Build history of the part. All positions in model axes, mm. Face numbers are marked on the shaded views. A direction names the side the tool comes from. Give positions to 0.01 mm unless a question says otherwise; leave off trailing zeros. Order: outer loops, then holes, each group sorted by start corner. A loop starts at its lowest first (then second) coordinate and runs counter-clockwise, first axis right, second up. Notation, with made-up numbers: (69, 32.5) -> (111, 32.5) arc R23 cw to (111, 48.5) -> close; hole circle Ø5 at (-25.75, -29). An arc over 180 degrees is marked (long way). One line per item, written item: value. Start each with the question number.
(1) Saw through at D-D on z = 5.25. Give the cut face in (x, y).
(2) Which spindle directions (+Z, -Z, +X, -X, +Y, -Y) get a long thin tool onto all of the face, cutting with end or side? Do the marked faces 5, 6, 7 and 8. Say none if no direction does.
(3) Saw through at C-C on z = -3. Give the cut face in (x, y), plus the area to 3 significant figures.
(4) Saw through at A-A on y = 0. Give the cut face in (x, z).
(5) Two-plate mould, pull along Y, no slides. Class the marked faces 1, 2, 3 and 4: +Y half, -Y half, draft (parallel to the pull), parting line (faces both ways), or undercut.
(6) Saw through at B-B on x = 0. Give the cut face in (y, z).
(7) Pin check, flat tips, straight feed: pin 1 (4 mm diameter, centred on y = 17, z = 5.5, fed in from -X); pin 2 (1.5 mm diameter, centred on x = 1, z = 6, fed in from +Y); pin 3 (1 mm diameter, centred on y = -15.5, z = -2.5, fed in from -X). Stop position of each tip, or through.
(8) Probe line 1 (X direction, y = -1, z = 5); line 2 (Y direction, x = 0, z = -0.75); line 3 (Z direction, x = -12.5, y = -17.5). List the from-to ranges inside material, lowest first.
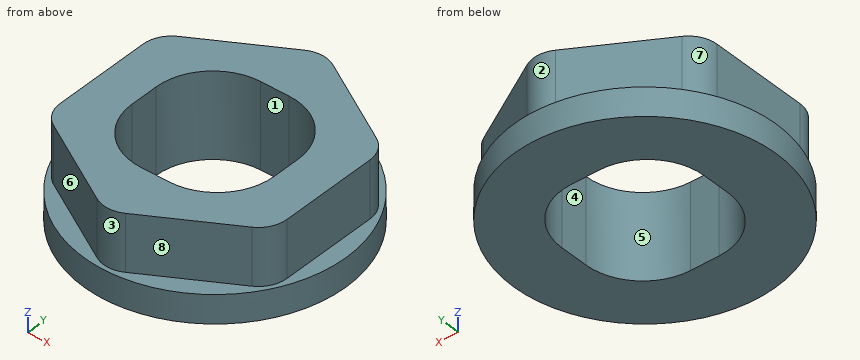
```python
from build123d import *

# Parameters (mm, degrees)
BOSS_EXTRUDE1_DEPTH = 10
SKETCH2_R           = 23.094010768
BOSS_EXTRUDE2_DEPTH = 5
FILLET1_R           = 5


with BuildPart() as part:
    # Sketch1 → Boss-Extrude1 (new body)
    with BuildSketch(Plane.XY):
        Polygon((20, -11.547005384), (20, 11.547005384), (0, 23.094010768), (-20, 11.547005384), (-20, -11.547005384), (0, -23.094010768), align=None)
        with BuildLine():
            Line((2.5, -12.5), (-2.5, -12.5))
            ThreePointArc((-2.5, -12.5), (-9.571067812, -9.571067812), (-12.5, -2.5))
            Line((-12.5, -2.5), (-12.5, 2.5))
            ThreePointArc((-12.5, 2.5), (-9.571067812, 9.571067812), (-2.5, 12.5))
            Line((-2.5, 12.5), (2.5, 12.5))
            ThreePointArc((2.5, 12.5), (9.571067812, 9.571067812), (12.5, 2.5))
            Line((12.5, 2.5), (12.5, -2.5))
            ThreePointArc((12.5, -2.5), (9.571067812, -9.571067812), (2.5, -12.5))
        make_face(mode=Mode.SUBTRACT)
    extrude(amount=BOSS_EXTRUDE1_DEPTH)

    # Sketch2 → Boss-Extrude2 (add)
    with BuildSketch(Plane(origin=(0, 0, 0), x_dir=(-1, 0, 0), z_dir=(0, 0, -1))):
        Circle(SKETCH2_R)
        with BuildLine():
            Line((-2.5, 12.5), (2.5, 12.5))
            ThreePointArc((2.5, 12.5), (9.571067812, 9.571067812), (12.5, 2.5))
            Line((12.5, 2.5), (12.5, -2.5))
            ThreePointArc((12.5, -2.5), (9.571067812, -9.571067812), (2.5, -12.5))
            Line((2.5, -12.5), (-2.5, -12.5))
            ThreePointArc((-2.5, -12.5), (-9.571067812, -9.571067812), (-12.5, -2.5))
            Line((-12.5, -2.5), (-12.5, 2.5))
            ThreePointArc((-12.5, 2.5), (-9.571067812, 9.571067812), (-2.5, 12.5))
        make_face(mode=Mode.SUBTRACT)
    extrude(amount=BOSS_EXTRUDE2_DEPTH)

    # Fillet1
    fillet1_edges = [part.edges().sort_by_distance(p)[0] for p in [
        (20, -11.547005384, 5),
        (0, -23.094010768, 5),
        (-20, -11.547005384, 5),
        (-20, 11.547005384, 5),
        (0, 23.094010768, 5),
        (20, 11.547005384, 5),
    ]]
    fillet(fillet1_edges, radius=FILLET1_R)


solid = part.part
```
Results below:
1. outline: (-20, -8.66) arc R5 ccw to (-17.5, -12.99) -> (-2.5, -21.65) arc R5 ccw to (2.5, -21.65) -> (17.5, -12.99) arc R5 ccw to (20, -8.66) -> (20, 8.66) arc R5 ccw to (17.5, 12.99) -> (2.5, 21.65) arc R5 ccw to (-2.5, 21.65) -> (-17.5, 12.99) arc R5 ccw to (-20, 8.66) -> close; hole (-12.5, -2.5) arc R10 ccw to (-2.5, -12.5) -> (2.5, -12.5) arc R10 ccw to (12.5, -2.5) -> (12.5, 2.5) arc R10 ccw to (2.5, 12.5) -> (-2.5, 12.5) arc R10 ccw to (-12.5, 2.5) -> close
2. face 5: +Z, -Z
2. face 6: +Z, -X, -Y
2. face 7: +Z, -X, +Y
2. face 8: +Z, +X, -Y
3. outline: circle Ø46.19 at (0, 0); hole (-12.5, -2.5) arc R10 ccw to (-2.5, -12.5) -> (2.5, -12.5) arc R10 ccw to (12.5, -2.5) -> (12.5, 2.5) arc R10 ccw to (2.5, 12.5) -> (-2.5, 12.5) arc R10 ccw to (-12.5, 2.5) -> close
3. area: 1,140 mm²
4. outline: (-23.09, -5) -> (-12.5, -5) -> (-12.5, 10) -> (-20, 10) -> (-20, 0) -> (-23.09, 0) -> close; (12.5, -5) -> (23.09, -5) -> (23.09, 0) -> (20, 0) -> (20, 10) -> (12.5, 10) -> close
5. face 1: undercut
5. face 2: +Y half
5. face 3: -Y half
5. face 4: undercut
6. outline: (-23.09, -5) -> (-12.5, -5) -> (-12.5, 10) -> (-22.32, 10) -> (-22.32, 0) -> (-23.09, 0) -> close; (12.5, -5) -> (23.09, -5) -> (23.09, 0) -> (22.32, 0) -> (22.32, 10) -> (12.5, 10) -> close
7. pin 1: stops at x = -14.02
7. pin 2: stops at y = 22.31
7. pin 3: stops at x = -17.56
8. line 1: x = -20 to -12.5, 12.5 to 20
8. line 2: y = -23.09 to -12.5, 12.5 to 23.09
8. line 3: z = -5 to 0
